```python
from build123d import *

# Parameters (mm, degrees)
CROQUIS1_R                       = 50
CROQUIS1_R_2                     = 15
SALIENTE_EXTRUIR1_DEPTH          = 15
CROQUIS2_R                       = 43.5
CROQUIS2_R_2                     = 15
SALIENTE_EXTRUIR2_DEPTH          = 8
CROQUIS3_R                       = 40
CROQUIS3_R_2                     = 15
SALIENTE_EXTRUIR3_DEPTH          = 4
TALADRO_DE_MARGEN_PARA_M31_D     = 3.4
TALADRO_DE_MARGEN_PARA_M31_DEPTH = 10
TALADRO_DE_MARGEN_PARA_M31_TIP   = 1.021463052
TALADRO_DE_MARGEN_PARA_M32_D     = 3.4
TALADRO_DE_MARGEN_PARA_M32_DEPTH = 20
TALADRO_DE_MARGEN_PARA_M32_TIP   = 1.021463052


with BuildPart() as part:
    # Croquis1 → Saliente-Extruir1 (new body)
    with BuildSketch(Plane(origin=(0, 0, 0), x_dir=(1, 0, 0), z_dir=(0, 1, 0))):
        with Locations(Location((0, 0, 0), (0, 0, 270))):
            Circle(CROQUIS1_R)
        with Locations(Location((0, 0, 0), (0, 0, 270))):
            Circle(CROQUIS1_R_2, mode=Mode.SUBTRACT)
    extrude(amount=SALIENTE_EXTRUIR1_DEPTH)

    # Croquis2 → Saliente-Extruir2 (add)
    with BuildSketch(Plane(origin=(0, 15, 0), x_dir=(1, 0, 0), z_dir=(0, 1, 0))):
        with Locations(Location((0, 0, 0), (0, 0, 270))):
            Circle(CROQUIS2_R)
        with Locations(Location((0, 0, 0), (0, 0, 270))):
            Circle(CROQUIS2_R_2, mode=Mode.SUBTRACT)
    extrude(amount=SALIENTE_EXTRUIR2_DEPTH)

    # Croquis3 → Saliente-Extruir3 (add)
    with BuildSketch(Plane(origin=(0, 23, 0), x_dir=(1, 0, 0), z_dir=(0, 1, 0))):
        with Locations(Location((0, 0, 0), (0, 0, 270))):
            Circle(CROQUIS3_R)
        with Locations(Location((0, 0, 0), (0, 0, 270))):
            Circle(CROQUIS3_R_2, mode=Mode.SUBTRACT)
    extrude(amount=SALIENTE_EXTRUIR3_DEPTH)

    # Taladro de margen para M31
    with Locations(Plane(origin=(0, 27, 0), x_dir=(1, 0, 0), z_dir=(0, 1, 0))):
        with Locations((0, 37.6), (26.587214973, 26.587214973), (37.6, 0), (26.587214973, -26.587214973), (0, -37.6), (-26.587214973, -26.587214973), (-37.6, 0), (-26.587214973, 26.587214973)):
            Hole(TALADRO_DE_MARGEN_PARA_M31_D / 2, depth=TALADRO_DE_MARGEN_PARA_M31_DEPTH)
            with Locations((0, 0, -(TALADRO_DE_MARGEN_PARA_M31_DEPTH + TALADRO_DE_MARGEN_PARA_M31_TIP / 2))):  # 118° drill point
                Cone(0, TALADRO_DE_MARGEN_PARA_M31_D / 2, TALADRO_DE_MARGEN_PARA_M31_TIP, mode=Mode.SUBTRACT)

    # Taladro de margen para M32
    with Locations(Plane(origin=(0, 27, 0), x_dir=(1, 0, 0), z_dir=(0, 1, 0))):
        with Locations((0, 25), (25, 0), (0, -25), (-25, 0)):
            Hole(TALADRO_DE_MARGEN_PARA_M32_D / 2, depth=TALADRO_DE_MARGEN_PARA_M32_DEPTH)
            with Locations((0, 0, -(TALADRO_DE_MARGEN_PARA_M32_DEPTH + TALADRO_DE_MARGEN_PARA_M32_TIP / 2))):  # 118° drill point
                Cone(0, TALADRO_DE_MARGEN_PARA_M32_D / 2, TALADRO_DE_MARGEN_PARA_M32_TIP, mode=Mode.SUBTRACT)


solid = part.part
```
Work out the finished part from the listing and answer in its coordinate system (mm). A direction names the side the tool comes from. Give positions to 0.01 mm unless a question says otherwise; leave off trailing zeros. Order: outer loops, then holes, each group sorted by start corner. A loop starts at its lowest first (then second) coordinate and runs counter-clockwise, first axis right, second up. Notation, with made-up numbers: M -33,38.25 L -7,38.25 A22 ccw -7,57.25 Z; hole C 7.5,4.5 d3. An arc over 180 degrees is marked long. Return JSON: item names as keys, results as strings.
1) Section D-D, the plane x = -20.5 is taken. Write down the section's boundary in (y, z), plus the area to 3 significant figures.
Resolved:
{"outline": "M 0,-45.6 L 15,-45.6 L 15,-38.37 L 23,-38.37 L 23,-34.35 L 27,-34.35 L 27,34.35 L 23,34.35 L 23,38.37 L 15,38.37 L 15,45.6 L 0,45.6 Z", "area": "2,260 mm^2"}
2) Section C-C, the plane z = 31 is taken. Write down the section's boundary in (x, y).
Resolved:
{"outline": "M -39.23,0 L 39.23,0 L 39.23,15 L 30.52,15 L 30.52,23 L 25.28,23 L 25.28,27 L -25.28,27 L -25.28,23 L -30.52,23 L -30.52,15 L -39.23,15 Z"}
3) Section A-A, the plane y = 11.5 is taken. Write down the section's boundary in (x, z).
Resolved:
{"outline": "C 0,0 d100; hole C -25,0 d3.4; hole C 0,0 d30; hole C 0,-25 d3.4; hole C 0,25 d3.4; hole C 25,0 d3.4"}
4) Straight lines are drawn through the part: line 1 along Z through (x, y) = (-1.5, 11); line 2 along Y through (x, z) = (37, 18); line 3 along Z through (x, y) = (-6.5, 10.5). For each, find the intervals that lie inside material, in ascending order. Write a range as [from, to].
Resolved:
{"line 1": "[-49.98, -25.8], [-24.2, -14.92], [14.92, 24.2], [25.8, 49.98]", "line 2": "[0, 23]", "line 3": "[-49.58, -13.52], [13.52, 49.58]"}
5) Each of these flat-tipped pins is pushed along its axis until it touches: pin 1 (3 mm diameter, centred on x = 37.6, z = 0, fed in from +Y); pin 2 (8 mm diameter, centred on y = 14.5, z = -1, fed in from +X); pin 3 (3 mm diameter, centred on x = 28.5, y = 15, fed in from -Z). Where does it stop, or does it pass through?
Resolved:
{"pin 1": "y = 16.88", "pin 2": "x = 50", "pin 3": "z = -42.08"}
6) A tool of negligible diameter and unlimited length cuts with its end or side. For faces 1 (the cylindrical face through (0.66, 13.311, -14.985)), 2 (the cylindrical face through (0.221, 16.86, -26.686)), from which of +Z, -Z, +X, -X, +Y, -Y can it reach the whole face along a straight path? Write none if from no direction.
Resolved:
{"face 1": "+Y, -Y", "face 2": "+Y"}
7) For a pull along X with two mould halves and no side action, classify faces 3 (the flat face through (12, 0, 10)), 4 (the conical face through (37.873, 16.156, 0.113)), 5 (the cylindrical face through (15.02, 7.4, 47.69)) as +X half, -X half, draft (parallel to the pull), parting line (faces both ways), or undercut.
Resolved:
{"face 3": "draft", "face 4": "undercut", "face 5": "parting line"}
8) Section B-B, the plane x = -8.5 is taken. Write down the section's boundary in (y, z).
Resolved:
{"outline": "M 0,-49.27 L 15,-49.27 L 15,-42.66 L 23,-42.66 L 23,-39.09 L 27,-39.09 L 27,-12.36 L 0,-12.36 Z; M 0,12.36 L 27,12.36 L 27,39.09 L 23,39.09 L 23,42.66 L 15,42.66 L 15,49.27 L 0,49.27 Z"}
